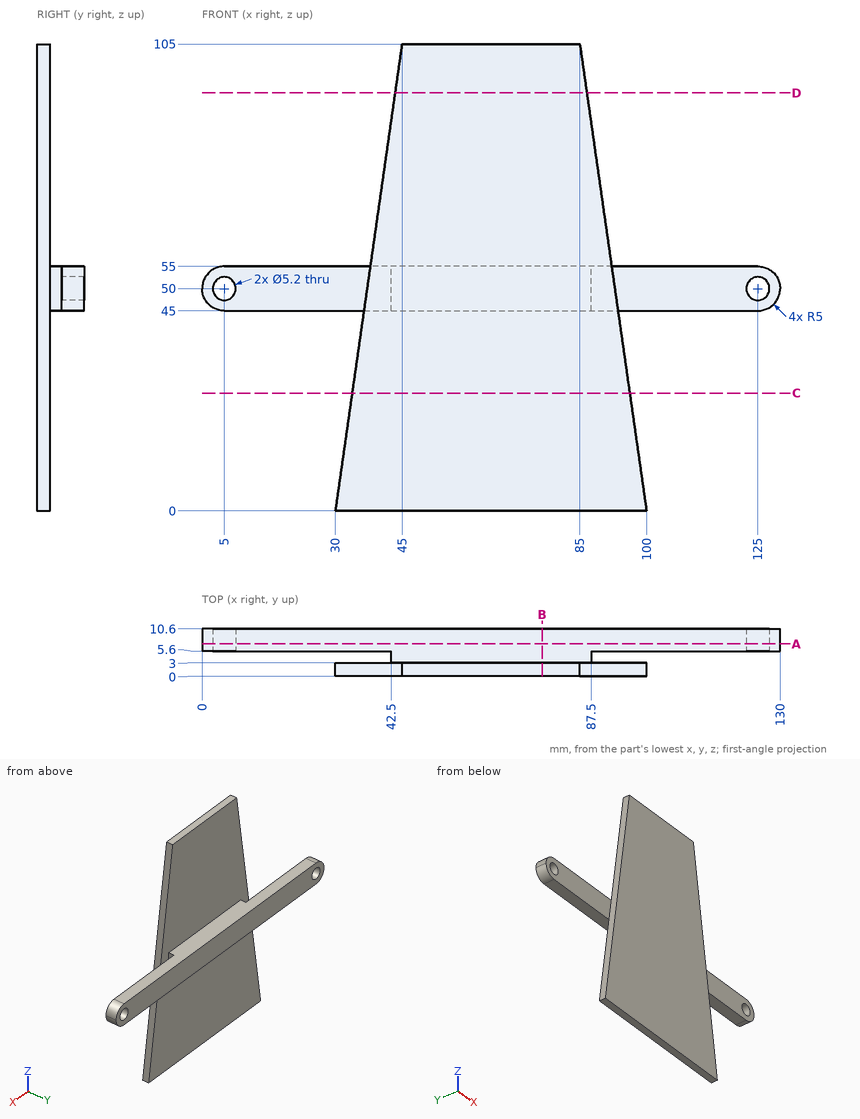
Can you work these out from the drawing? Everything is in mm from the part's minimum corner. Round coordinates to 2 decimals unless told otherwise and drop trailing zeros. Loops run counter-clockwise (first coordinate to the right, second up) from the corner with the lowest first, then second, coordinate; pieces in that order, holes last. Notation, with made-up numbers: (29, 78) - (62, 78) arc R12 ccw to (62, 96) - close; hole circle Ø5 at (19, 22.5). An arc over 180 degrees is marked (long way). Write item = value, one per line. Start each with the question number.
(1) If we section it at D-D (z = 94): Please give me the cut outline in (x, y), and give its area (3 significant figures).
(2) If I drill on probe 1 along X at (y, z) = (7.55, 50); probe 2 along Z at (x, y) = (5, 9.2); probe 3 along Y at (x, z) = (51.5, 64), over which ranges is the centre line in solid material (lowest first)? Write a range as [from, to].
(3) If we section it at A-A (y = 7.25): Give the number of separate pieces and of enclosed holes in the cut face, and give its area (3 significant figures).
(4) If we section it at C-C (z = 26.5): Please give me the cut outline in (x, y).
(5) If we section it at B-B (x = 76.5): Please give me the cut outline in (y, z), and give its area (3 significant figures).
(6) For P1, Ø1, axis at y = 4, z = 85, coming from the +X side; P2, Ø8, axis at x = 100, z = 48.5, coming from the -Y side; P3, Ø0.8, axis at y = 4, z = 50, coming from the +X side; P4, Ø1.5, axis at x = 102.5, y = 8.5, coming from the +Z side, each with a flat end and sliding along its axis, tell me the tip position at first contact or that it passes through.
Ans:
q1.outline = (43.43, 0) - (86.57, 0) - (86.57, 3) - (43.43, 3) - close
q1.area = 129 mm²
q2.probe_1 = [0, 2.4], [7.6, 122.4], [127.6, 130]
q2.probe_2 = [45, 47.4], [52.6, 55]
q2.probe_3 = [0, 3]
q3.separate_pieces = 1
q3.enclosed_holes = 2
q3.area = 1,240 mm²
q4.outline = (33.79, 0) - (96.21, 0) - (96.21, 3) - (33.79, 3) - close
q5.outline = (0, 0) - (3, 0) - (3, 45) - (10.6, 45) - (10.6, 55) - (3, 55) - (3, 105) - (0, 105) - close
q5.area = 391 mm²
q6.P1 = through
q6.P2 = 5.6
q6.P3 = 87.5
q6.P4 = 55
